```python
from build123d import *


with BuildPart() as part:
    # Sketch1 → Revolve1 (revolve)
    with BuildSketch(Plane(origin=(0, 0, 0), x_dir=(-1, 0, 0), z_dir=(0, 0, -1)), mode=Mode.PRIVATE) as revolve1_sk:
        with BuildLine():
            Line((5.84, 4), (-5.84, 4))
            ThreePointArc((-5.84, 4), (-5.953137085, 3.953137085), (-6, 3.84))
            Line((-6, 3.84), (-6, 3.36))
            Line((-6, 3.36), (-5.88, 3.36))
            Line((-5.88, 3.36), (-5.88, 2))
            Line((-5.88, 2), (5.88, 2))
            Line((5.88, 2), (5.88, 3.36))
            Line((5.88, 3.36), (6, 3.36))
            Line((6, 3.36), (6, 3.84))
            ThreePointArc((6, 3.84), (5.953137085, 3.953137085), (5.84, 4))
        make_face()
    revolve(revolve1_sk.sketch.rotate(Axis((6, 0, 0), (-1, 0, 0)), 270), axis=Axis((6, 0, 0), (-1, 0, 0)))


solid = part.part
```
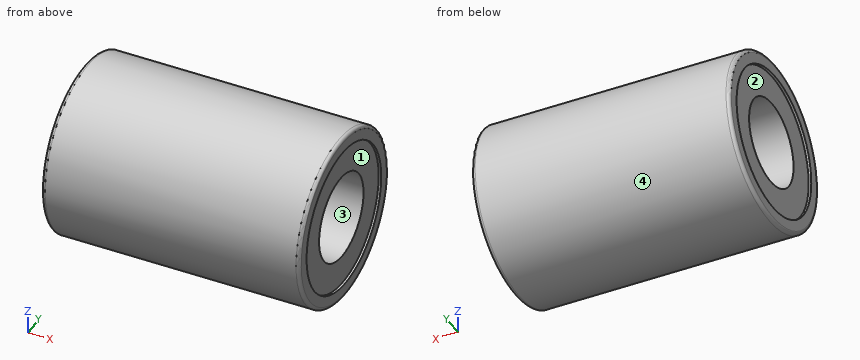
Check sheet for the modelled part. Datum: model origin and axes. Units: mm. Face numbers are marked on the shaded views. A direction names the side the tool comes from. Round coordinates to 2 decimals unless told otherwise and drop trailing zeros. Loops run counter-clockwise (first coordinate to the right, second up) from the corner with the lowest first, then second, coordinate; pieces in that order, holes last. Notation, with made-up numbers: M 87,88 L 111,88 A27 ccw 111,119 Z; hole C 76.5,58.25 d6. An arc over 180 degrees is marked long. Answer as a JSON object with one key per item and string values.
1. Gauge pin test, flat ends, axial feed: P1, Ø2, axis at y = 0, z = -1.5, coming from the +X side; P2, Ø3.5, axis at y = 0, z = 0, coming from the +X side; P3, Ø1.5, axis at x = 0.5, z = -1.5, coming from the -Y side; P4, Ø1, axis at x = -2.5, z = -1, coming from the -Y side. Record the tip position at first contact, or that the pin passes through.
Reply:
{"P1": "stops at x = 5.88", "P2": "passes through", "P3": "stops at y = -3.93", "P4": "stops at y = -3.97"}
2. Mould release check, pull along Z, two halves, no side actions. Record for the marked faces 3 and 4: pulls with the +Z half, pulls with the -Z half, needs draft (parallel to the pull), parting line crosses it, or undercut.
Reply:
{"face 3": "undercut", "face 4": "parting line crosses it"}
3. Scan lines: line 1 (Y direction, x = 1.25, z = 0); line 2 (Y direction, x = 5, z = 0.75); line 3 (X direction, y = -2.5, z = 0). Record each from-to range of solid material in increasing order.
Reply:
{"line 1": "y = -4 to -2, 2 to 4", "line 2": "y = -3.93 to -1.85, 1.85 to 3.93", "line 3": "x = -5.88 to 5.88"}
4. Access from +Z, -Z, +X, -X, +Y, -Y to the whole of each face (thin tool, end or side, straight path). Record for the marked faces 1 and 2.
Reply:
{"face 1": "+X", "face 2": "-X"}
5. Section check C-C (x = 2). Record the boundary of the cut face in (y, z).
Reply:
{"outline": "C 0,0 d8; hole C 0,0 d4"}
6. Section check A-A (z = 0). Record the boundary of the cut face in (x, y).
Reply:
{"outline": "M -6,-3.84 A0.16 ccw -5.84,-4 L 5.84,-4 A0.16 ccw 6,-3.84 L 6,-3.36 L 5.88,-3.36 L 5.88,-2 L -5.88,-2 L -5.88,-3.36 L -6,-3.36 Z; M -6,3.36 L -5.88,3.36 L -5.88,2 L 5.88,2 L 5.88,3.36 L 6,3.36 L 6,3.84 A0.16 ccw 5.84,4 L -5.84,4 A0.16 ccw -6,3.84 Z"}
